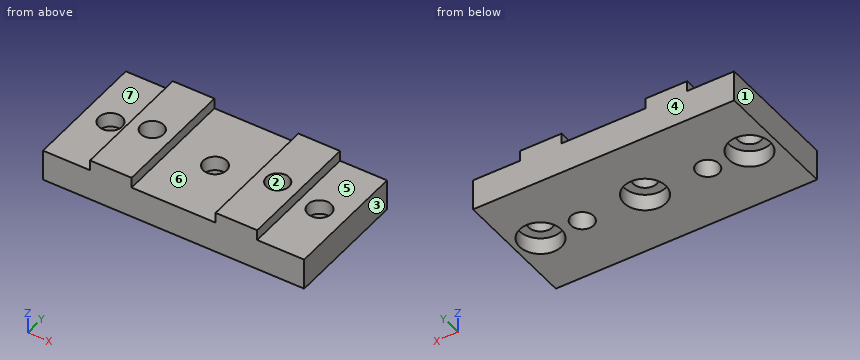
```python
from build123d import *

# Parameters (mm, degrees)
SKETCH1_W             = 39.6748
SKETCH1_H             = 19.05
EXTRUDE1_DEPTH        = 6.35
SKETCH2_W             = 7.1374
SKETCH2_H             = 1.6002
SKETCH2_W_2           = 12.7508
CUT_EXTRUDE1_DEPTH    = 20.05
HOLE1_D               = 3.556
HOLE1_CBORE_D         = 6.35
HOLE1_CBORE_DEPTH     = 2.54
F_8_32_TAPPED_HOLE1_D = 3.4544


with BuildPart() as part:
    # Sketch1 → Extrude1 (new body)
    with BuildSketch(Plane.XY):
        with Locations((19.8374, 9.525)):
            Rectangle(SKETCH1_W, SKETCH1_H)
    extrude(amount=EXTRUDE1_DEPTH)

    # Sketch2 → Cut-Extrude1 (cut, through all)
    with BuildSketch(Plane.XZ):
        with Locations((3.5687, 5.5499)):
            Rectangle(SKETCH2_W, SKETCH2_H)
        with Locations((19.8374, 5.5499)):
            Rectangle(SKETCH2_W_2, SKETCH2_H)
        with Locations((36.1061, 5.5499)):
            Rectangle(SKETCH2_W, SKETCH2_H)
    extrude(amount=-CUT_EXTRUDE1_DEPTH, mode=Mode.SUBTRACT)

    # Hole1 (through all)
    with Locations(Plane(origin=(0, 0, 0), x_dir=(-1, 0, 0), z_dir=(0, 0, -1))):
        with Locations((-3.9624, 9.525), (-19.8374, 9.525), (-35.7124, 9.525)):
            CounterBoreHole(HOLE1_D / 2, HOLE1_CBORE_D / 2, HOLE1_CBORE_DEPTH)

    # #8-32 Tapped Hole1 (through all)
    with Locations(Plane(origin=(0, 0, 0), x_dir=(-1, 0, 0), z_dir=(0, 0, -1))):
        with Locations((-10.3124, 9.525), (-29.3624, 9.525)):
            Hole(F_8_32_TAPPED_HOLE1_D / 2)


solid = part.part
```
For this review, take the finished solid that the model builds, in its own axes (mm). Face numbers are marked on the shaded views. A direction names the side the tool comes from. Give positions to 0.01 mm unless a question says otherwise; leave off trailing zeros. Write each loop counter-clockwise with the first axis right and the second up, starting at its lowest first coordinate (ties: lowest second). Pieces come first, ordered by that corner, then holes. Notation, with made-up numbers: M -32.75,51.5 L -19.75,51.5 A23 cw -19.75,81.5 Z; hole C 38.25,0 d7. An arc over 180 degrees is marked long. Answer as a JSON object with one key per item and string values. Group by question number.
Item 1: Consider section A-A on x = 4. Write out the cut boundary in (y, z).
Item 2: For probe 1 along X at (y, z) = (9.5, 6); probe 2 along X at (y, z) = (9, 1.5); probe 3 along X at (y, z) = (6.5, 6), list the stretches that pass through material, from the lowest coordinate up. Write a range as [from, to].
Item 3: Consider section D-D on x = 36. Write out the cut boundary in (y, z), plus the area to 3 significant figures.
Item 4: Tool access review of the marked faces 5, 6 and 7: name each direction out of +Z, -Z, +X, -X, +Y, -Y from which nothing blocks a thin tool from reaching the whole face with its end or side.
Item 5: Draft analysis for pull direction X (two halves, no side actions). For the marked faces 1, 2, 3 and 4, state which applies: +X half, -X half, draft (parallel to the pull), parting line (faces both ways), or undercut.
Item 6: Consider section C-C on y = 18. Write out the cut boundary in (x, z).
Item 7: For pin 1 Ø0.5 at (y, z) = (5, 6) entering from -X; pin 2 Ø6 at (x, y) = (19, 16.5) entering from +Z; pin 3 Ø3 at (x, y) = (4.5, 9) entering from -Z, all flat-tipped, find the tip position at first contact; note any pin that passes through.
Item 8: Consider section B-B on z = 3.5. Write out the cut boundary in (x, y) (3 decimals).
Check result:
{
 "1": {"outline": "M 0,0 L 6.35,0 L 6.35,2.54 L 7.75,2.54 L 7.75,4.75 L 0,4.75 Z; M 11.3,2.54 L 12.7,2.54 L 12.7,0 L 19.05,0 L 19.05,4.75 L 11.3,4.75 Z"},
 "2": {"probe 1": "x = [7.14, 8.59], [12.04, 13.46], [26.21, 27.64], [31.09, 32.54]", "probe 2": "x = [0, 0.83], [7.09, 8.67], [11.96, 16.71], [22.97, 27.72], [31.01, 32.58], [38.84, 39.67]", "probe 3": "x = [7.14, 13.46], [26.21, 32.54]"},
 "3": {"outline": "M 0,0 L 6.36,0 L 6.36,2.54 L 7.77,2.54 L 7.77,4.75 L 0,4.75 Z; M 11.28,2.54 L 12.69,2.54 L 12.69,0 L 19.05,0 L 19.05,4.75 L 11.28,4.75 Z", "area": "66.7 mm^2"},
 "4": {"face 5": "+Z, +X, +Y, -Y", "face 6": "+Z, +Y, -Y", "face 7": "+Z, -X, +Y, -Y"},
 "5": {"face 1": "-X half", "face 2": "undercut", "face 3": "+X half", "face 4": "draft"},
 "6": {"outline": "M 0,0 L 39.67,0 L 39.67,4.75 L 32.54,4.75 L 32.54,6.35 L 26.21,6.35 L 26.21,4.75 L 13.46,4.75 L 13.46,6.35 L 7.14,6.35 L 7.14,4.75 L 0,4.75 Z"},
 "7": {"pin 1": "stops at x = 7.14", "pin 2": "stops at z = 4.75", "pin 3": "stops at z = 2.54"},
 "8": {"outline": "M 0,0 L 39.675,0 L 39.675,19.05 L 0,19.05 Z; hole C 3.962,9.525 d3.556; hole C 10.312,9.525 d3.454; hole C 19.837,9.525 d3.556; hole C 29.362,9.525 d3.454; hole C 35.712,9.525 d3.556"}
}
